Autodesk Fusion 360 part; units mm, degrees
sketch "Sketch1" plane through (0, 0, 0) normal (0, 0, 1) x (1, 0, 0)
  line L0 (-45, -42) -> (-45, -38)
  line L1 (-45, -38) -> (-30, -38)
  line L2 (-30, -38) -> (-30, 8)
  line L3 (-30, 8) -> (30, 8)
  line L4 (30, 8) -> (30, -38)
  line L5 (30, -38) -> (45, -38)
  line L6 (45, -38) -> (45, -42)
  line L7 (45, -42) -> (25, -42)
  line L8 (25, -42) -> (25, -2)
  line L9 (25, -2) -> (-25, -2)
  line L10 (-25, -2) -> (-25, -42)
  line L11 (-25, -42) -> (-45, -42)
  dimension "d1" = 60
  dimension "d2" = 30
  dimension "d3" = 4
  dimension "d4" = 4
  dimension "d5" = 5
  dimension "d6" = 5
  dimension "d7" = 10
  dimension "d8" = 15
  dimension "d9" = 15
  dimension "d24" = 46
  dimension "d25" = 46
extrude "Extrude1" add sketch "Sketch1" along normal blind 60
sketch "Sketch2" plane through (0, 8, 0) normal (0, 1, 0) x (-1, 0, 0)
  line L0 (-30, 0) -> (30, 0)
  line L1 (30, 0) -> (30, 60)
  line L2 (30, 60) -> (-30, 60)
  line L3 (-30, 60) -> (-30, 0)
  circle A0 centre (0, 30) radius 21.1
  dimension "d14" = 42.2
  dimension "d15" = 30
  dimension "d16" = 30
extrude "Extrude2" cut sketch "Sketch2" against normal blind 7 contours A0
sketch "Sketch3" plane through (0, 1, 0) normal (0, 1, 0) x (-1, 0, 0)
  circle A0 centre (0, 30) radius 21.1
  circle A1 centre (0, 30) radius 19
  dimension "d20" = 38
extrude "Extrude3" cut sketch "Sketch3" against normal up to surface (3 mm away) contours A1
chamfer "Chamfer1" distance 10 distance2 15 1 edges at (-30, -38, 30) measured on face at (-30, -22.6667, 40)
chamfer "Chamfer2" distance 15 distance2 10 1 edges at (30, -38, 30) measured on face at (35, -38, 20)
chamfer "Chamfer3" distance 1.5 angle 45 1 edges at (19.6721, 8, 37.6301)
chamfer "Chamfer4" distance 2 distance2 1 2 edges at (0, 8, 0) (0, 8, 60) measured on face at (33.3323, -36.0007, 0) measured on face at (33.3323, -36.0007, 60)
chamfer "Chamfer5" distance 2 distance2 1 1 edges at (30, 8, 30) measured on face at (30, -5.334, 40)
chamfer "Chamfer6" distance 1 distance2 2 1 edges at (-30, 8, 30) measured on face at (-27.5333, 8, 30)
chamfer "Chamfer7" distance 3 angle 45 2 edges at (25, -2, 30) (-25, -2, 30)
sketch "Sketch4" plane through (0, 8, 0) normal (0, 1, 0) x (-1, 0, 0)
  circle A0 centre (0, 30) radius 22.6
  line L0 (29, 1) -> (29, 59)
  line L1 (29, 59) -> (-29, 59)
  line L2 (-29, 59) -> (-29, 1)
  line L3 (-29, 1) -> (29, 1)
  circle A1 centre (-19.5, 10.5) radius 1.65
  circle A2 centre (19.5, 10.5) radius 1.65
  circle A3 centre (19.5, 49.5) radius 1.65
  circle A4 centre (-19.5, 49.5) radius 1.65
  dimension "d40" = 3.3
  dimension "d41" = 19.5
  dimension "d42" = 19.5
  dimension "d44" = 360
extrude "Extrude4" cut sketch "Sketch4" against normal blind 15 contours A1 | A2 | A3 | A4
sketch "Sketch5" plane through (0, -2, 0) normal (0, -1, 0) x (1, 0, 0)
  circle A0 centre (-19.5, 10.5) radius 1.65
  circle A1 centre (-19.5, 49.5) radius 1.65
  circle A2 centre (19.5, 10.5) radius 1.65
  circle A3 centre (19.5, 49.5) radius 1.65
  circle A4 centre (0, 30) radius 19
  line L0 (-22, 60) -> (-22, 0)
  line L1 (-22, 0) -> (22, 0)
  line L2 (22, 0) -> (22, 60)
  line L3 (22, 60) -> (-22, 60)
  circle A5 centre (19.5, 49.5) radius 4
  circle A6 centre (-19.5, 49.5) radius 4
  circle A7 centre (-19.5, 10.5) radius 4
  circle A8 centre (19.5, 10.5) radius 4
  dimension "d47" = 8
  dimension "d49" = 360
extrude "Extrude5" cut sketch "Sketch5" along normal blind -2 and the other way blind -2 contours L0 A6 | L0 A6 | L2 A5 | L2 A5 | L0 A7 | L0 A7 | L2 A8 | L2 A8
sketch "Sketch6" plane through (0, -42, 0) normal (0, -1, 0) x (1, 0, 0)
  line L0 (25, 0) -> (45, 0)
  line L1 (45, 0) -> (45, 60)
  line L2 (45, 60) -> (25, 60)
  line L3 (25, 60) -> (25, 0)
  circle A0 centre (35.5, 50) radius 1.65
  circle A1 centre (35.5, 10) radius 1.65
  circle A2 centre (-35.5, 10) radius 1.65
  circle A3 centre (-35.5, 50) radius 1.65
  arc A4 (-22, 46.3775) -> (-22, 52.6225) centre (-19.5, 49.5) ccw
  arc A5 (22, 52.6225) -> (22, 46.3775) centre (19.5, 49.5) ccw
  arc A6 (22, 13.6225) -> (22, 7.3775) centre (19.5, 10.5) ccw
  arc A7 (-22, 7.3775) -> (-22, 13.6225) centre (-19.5, 10.5) ccw
  dimension "d54" = 3.3
  dimension "d55" = 10
  dimension "d57" = 3.3
  dimension "d59" = 10
  dimension "d60" = 3.3
  dimension "d61" = 10
  dimension "d63" = 3.3
  dimension "d64" = 10
  dimension "d66" = 16
  dimension "d67" = 16
  dimension "d68" = 16
  dimension "d69" = 16
extrude "Extrude6" cut sketch "Sketch6" against normal blind 25 contours A0 | A1 | A2 | A3
sketch "Sketch7" plane through (45, 0, 0) normal (1, 0, 0) x (0, 0, -1)
  line L0 (0, -42) -> (0, -38)
  line L1 (0, -38) -> (-60, -38)
  line L2 (-60, -38) -> (-60, -42)
  line L3 (-60, -42) -> (0, -42)
  line L4 (-54, -28) -> (-46, -28)
  line L5 (-46, -28) -> (-46, -34)
  line L6 (-46, -34) -> (-54, -34)
  line L7 (-54, -34) -> (-54, -28)
  line L8 (-14, -28) -> (-6, -28)
  line L9 (-6, -28) -> (-6, -34)
  line L10 (-6, -34) -> (-14, -34)
  line L11 (-14, -34) -> (-14, -28)
  dimension "d72" = 8
  dimension "d73" = 6
  dimension "d74" = 8
  dimension "d75" = 8
  dimension "d76" = 8
  dimension "d77" = 6
extrude "Extrude7" cut sketch "Sketch7" against normal blind 15 contours L4 L5 L6 L7 | L8 L9 L10 L11
sketch "Sketch8" plane through (-45, 0, 0) normal (-1, 0, 0) x (0, 0, 1)
  line L0 (0, -38) -> (0, -42)
  line L1 (0, -42) -> (60, -42)
  line L2 (60, -42) -> (60, -38)
  line L3 (60, -38) -> (0, -38)
  line L4 (6, -28) -> (14, -28)
  line L5 (14, -28) -> (14, -34)
  line L6 (14, -34) -> (6, -34)
  line L7 (6, -34) -> (6, -28)
  line L8 (46, -28) -> (54, -28)
  line L9 (54, -28) -> (54, -34)
  line L10 (54, -34) -> (46, -34)
  line L11 (46, -34) -> (46, -28)
  dimension "d80" = 8
  dimension "d81" = 8
  dimension "d82" = 6
  dimension "d83" = 8
  dimension "d84" = 8
  dimension "d85" = 6
extrude "Extrude8" cut sketch "Sketch8" against normal blind 15 contours L4 L5 L6 L7 | L8 L9 L10 L11
fillet "Fillet1" radius 5 4 edges at (-45, -40, 0) (45, -40, 0) (45, -40, 60) (-45, -40, 60)
sketch "Sketch9" plane through (30, 0, 0) normal (1, 0, 0) x (0, 0, -1)
  line L0 (0, 6) -> (-60, 6)
  line L1 (-60, 6) -> (-60, -28)
  line L2 (-60, -28) -> (-54, -28)
  line L3 (-54, -28) -> (-54, -34)
  line L4 (-54, -34) -> (-46, -34)
  line L5 (-46, -34) -> (-46, -28)
  line L6 (-46, -28) -> (-14, -28)
  line L7 (-14, -28) -> (-14, -34)
  line L8 (-14, -34) -> (-6, -34)
  line L9 (-6, -34) -> (-6, -28)
  line L10 (-6, -28) -> (0, -28)
  line L11 (0, -28) -> (0, 6)
  line L12 (-45, -20) -> (-15, -20)
  arc A0 (-15, -20) -> (-15, -10) centre (-15, -15) ccw
  line L13 (-15, -10) -> (-45, -10)
  arc A1 (-45, -10) -> (-45, -20) centre (-45, -15) ccw
  line L14 (-45, -15) -> (-15, -15) construction
  dimension "d89" = 30
  dimension "d90" = 15
  dimension "d91" = 15
extrude "Extrude9" cut sketch "Sketch9" against normal up to surface (60 mm away) contours L12 A0 L13 A1
equation "d1 = main"
equation "d2 = d1 / 2"
equation "d3 = leg_thickness"
equation "d4 = leg_thickness"
equation "d6 = d5"
equation "d8 = leg"
equation "d9 = leg"
equation "main = 60 mm"
equation "d11 = main"
equation "bearing_od = 42.2 mm"
equation "d14 = bearing_od"
equation "d15 = main / 2"
equation "d16 = main / 2"
equation "bearing_thickness = 7 mm"
equation "height = 46 mm"
equation "d24 = height"
equation "d25 = height"
equation "leg = 15 mm"
equation "d28 = leg"
equation "d29 = leg"
equation "leg_thickness = 4 mm"
equation "d41 = d42"
equation "d57 = d54"
equation "d59 = d55"
equation "d60 = d54"
equation "d61 = d55"
equation "d63 = d54"
equation "d64 = d55"
equation "d66 = d67"
equation "d68 = d67"
equation "d69 = d67"
equation "d75 = d72"
equation "d76 = d74"
equation "d77 = d73"
Model file for the job. Use its own axes, mm. A direction names the side the tool comes from. Round coordinates to 2 decimals unless told otherwise and drop trailing zeros. Loops run counter-clockwise (first coordinate to the right, second up) from the corner with the lowest first, then second, coordinate; pieces in that order, holes last. Notation, with made-up numbers: M -9.75,-16 L 10.25,-16 A33 ccw 10.25,20 Z; hole C 24.25,56.25 d5. An arc over 180 degrees is marked long. One line per question, with ' | ' between items.
1) Band-saw the part on B-B (x = 0). Give the cut face in (y, z).
Solved:
outline: M -2,0 L 6,0 L 8,1 L 8,7.4 L 6.5,8.9 L 1,8.9 L 1,11 L -2,11 Z; M -2,49 L 1,49 L 1,51.1 L 6.5,51.1 L 8,52.6 L 8,59 L 6,60 L -2,60 Z
2) Flat gauge pins, fed straight in: pin 1 (12 mm diameter, centred on y = -6.5, z = 17, fed in from +X); pin 2 (4 mm diameter, centred on y = -5.5, z = 46.5, fed in from -X); pin 3 (6.5 mm diameter, centred on x = 33, z = 51, fed in from +Y). Where does each tip first touch, or does it go through?
Solved:
pin 1: stops at x = 30 | pin 2: stops at x = -30 | pin 3: stops at y = 6.5
3) Drill centre lines: line 1 along Z through (x, y) = (19.5, -0.7); line 2 along Z through (x, y) = (35.5, -39.5); line 3 along X through (y, z) = (-26, 31.5). Where is each one in solid material? Low to high.
Solved:
line 1: z = 0 to 6.5, 14.5 to 45.5, 53.5 to 60 | line 2: z = 0 to 8.35, 11.65 to 48.35, 51.65 to 60 | line 3: x = -30 to -25, 25 to 30
4) Band-saw the part on A-A (y = 4). Give the cut face in (x, z).
Solved:
outline: M -30,0 L 30,0 L 30,60 L -30,60 Z; hole C -19.5,10.5 d3.3; hole C -19.5,49.5 d3.3; hole C 0,30 d42.2; hole C 19.5,10.5 d3.3; hole C 19.5,49.5 d3.3
5) Band-saw the part on D-D (y = -23). Give the cut face in (x, z), then the cut area to 3 significant figures.
Solved:
outline: M -30,0 L -25,0 L -25,60 L -30,60 Z; M 25,0 L 30,0 L 30,60 L 25,60 Z | area: 600 mm²
6) Band-saw the part on C-C (y = -15). Give the cut face in (x, z), then the cut area to 3 significant figures.
Solved:
outline: M -30,0 L -25,0 L -25,10 L -30,10 Z; M -30,50 L -25,50 L -25,60 L -30,60 Z; M 25,0 L 30,0 L 30,10 L 25,10 Z; M 25,50 L 30,50 L 30,60 L 25,60 Z | area: 200 mm²
7) Mould opens along Z. For faces 1 (the flat face through (-37.6, -33.07, 29.58)), 2 (the flat face through (-0.4, 7, 0.5)), 3 (the flat face through (-33, -32, 46)) say: +Z half, -Z half, draft (parallel to the pull), parting line (faces both ways), or undercut.
Solved:
face 1: draft | face 2: -Z half | face 3: undercut
8) 3-axis set-ups, long thin cutter, end or side, ignore diameter. For faces 4 (the cylindrical face through (-27, -15, 50)), 5 (the flat face through (-17.8, 0, 48.7)), 6 (the cylindrical face through (2.75, 3.79, 50.92)): which of +Z, -Z, +X, -X, +Y, -Y reach the whole face in a straight line?
Solved:
face 4: +X, -X | face 5: -Y | face 6: +Y
